Here's how the part is built. I have some questions about the finished solid (model axes, mm). A direction names the side the tool comes from. Round coordinates to 2 decimals unless told otherwise and drop trailing zeros. Order: outer loops, then holes, each group sorted by start corner. A loop starts at its lowest first (then second) coordinate and runs counter-clockwise, first axis right, second up.
```python
from build123d import *

# Parameters (mm, degrees)
SKETCH_1_W          = 10
SKETCH_1_H          = 10
SKETCH_1_W_2        = 8
SKETCH_1_H_2        = 8
EXTRUDE_1_DEPTH     = 75
SKETCH_2_R          = 2.15
CUT_EXTRUDE_1_DEPTH = 76.828754441
SKETCH_3_R          = 2.15
CUT_EXTRUDE_2_DEPTH = 76.828754441


with BuildPart() as part:
    # ｽｹｯﾁ1 → 押し出し-薄板1 (new body)
    with BuildSketch(Plane(origin=(0, 0, 0), x_dir=(0, 0, -1), z_dir=(1, 0, 0))):
        Rectangle(SKETCH_1_W, SKETCH_1_H)
        Rectangle(SKETCH_1_W_2, SKETCH_1_H_2, mode=Mode.SUBTRACT)
    extrude(amount=EXTRUDE_1_DEPTH)

    # ｽｹｯﾁ2 → ｶｯﾄ - 押し出し1 (cut, through all)
    with BuildSketch(Plane.XY.offset(5)):
        with Locations((70, 0)):
            Circle(SKETCH_2_R)
        with Locations(Location((5, 0, 0), (0, 0, 90))):
            Circle(SKETCH_2_R)
    extrude(amount=-CUT_EXTRUDE_1_DEPTH, mode=Mode.SUBTRACT)

    # ｽｹｯﾁ3 → ｶｯﾄ - 押し出し2 (cut, through all)
    with BuildSketch(Plane(origin=(0, 5, 0), x_dir=(1, 0, 0), z_dir=(0, 1, 0))):
        with Locations(Location((42.5, 0, 0), (0, 0, 270))):
            Circle(SKETCH_3_R)
        with Locations(Location((32.5, 0, 0), (0, 0, 270))):
            Circle(SKETCH_3_R)
    extrude(amount=-CUT_EXTRUDE_2_DEPTH, mode=Mode.SUBTRACT)


solid = part.part
```
1. If we section it at B-B, the plane y = 3: Write out the boundary of the cut face in (x, z).
Evaluation:
outline: (0, -5) - (75, -5) - (75, -4) - (0, -4) - close; (0, 4) - (75, 4) - (75, 5) - (0, 5) - close
2. If we mould it in two halves opening along Z, with no side actions, what happens to faces 3 (the flat face through (37, 0, -5)), 4 (the flat face through (37, -5, 0)), 5 (the flat face through (37, 4, 0))? For each: released by +Z, released by -Z, zero draft, split by the parting line, or undercut.
Evaluation:
face 3: released by -Z
face 4: zero draft
face 5: undercut
3. On a 3-axis mill with a long thin cutter (end or side, diameter ignored), from which of +Z, -Z, +X, -X, +Y, -Y can I reach the whole of each face in a straight line? I mean faces 1 (the flat face through (37, 0, -4)), 2 (the cylindrical face through (44.63, 4.51, -0.28)). Say none if no direction works.
Evaluation:
face 1: +X, -X
face 2: +Y, -Y
4. If we section it at D-D, the plane y = 0: Write out the boundary of the cut face in (x, z), and give its area (3 significant figures).
Evaluation:
outline: (0, -5) - (2.85, -5) - (2.85, -4) - (0, -4) - close; (0, 4) - (2.85, 4) - (2.85, 5) - (0, 5) - close; (7.15, -5) - (67.85, -5) - (67.85, -4) - (7.15, -4) - close; (7.15, 4) - (67.85, 4) - (67.85, 5) - (7.15, 5) - close; (72.15, -5) - (75, -5) - (75, -4) - (72.15, -4) - close; (72.15, 4) - (75, 4) - (75, 5) - (72.15, 5) - close
area: 133 mm2
5. If we section it at C-C, the plane x = 42.5: Write out the boundary of the cut face in (y, z), and give its area (3 significant figures).
Evaluation:
outline: (-5, -5) - (5, -5) - (5, -2.15) - (4, -2.15) - (4, -4) - (-4, -4) - (-4, -2.15) - (-5, -2.15) - close; (-5, 2.15) - (-4, 2.15) - (-4, 4) - (4, 4) - (4, 2.15) - (5, 2.15) - (5, 5) - (-5, 5) - close
area: 27.4 mm2
6. If we section it at A-A, the plane z = 0: Write out the boundary of the cut face in (x, y).
Evaluation:
outline: (0, -5) - (30.35, -5) - (30.35, -4) - (0, -4) - close; (0, 4) - (30.35, 4) - (30.35, 5) - (0, 5) - close; (34.65, -5) - (40.35, -5) - (40.35, -4) - (34.65, -4) - close; (34.65, 4) - (40.35, 4) - (40.35, 5) - (34.65, 5) - close; (44.65, -5) - (75, -5) - (75, -4) - (44.65, -4) - close; (44.65, 4) - (75, 4) - (75, 5) - (44.65, 5) - close
7. I need wall thicknesses on probe 1 along X at (y, z) = (4.65, 0); probe 2 along Z at (x, y) = (40.5, 2). Which ranges of each line are inside material? Lowest first, please.
Evaluation:
probe 1: x = 0 to 30.35, 34.65 to 40.35, 44.65 to 75
probe 2: z = -5 to -4, 4 to 5
